The figure shows three views and two pictorial views of one solid part (mm, origin at its lowest corner). Answer the questions. Coordinates: 2 decimals unless noted, no trailing zeros. Order: outer loops, then holes, each group sorted by start corner. A loop starts at its lowest first (then second) coordinate and runs counter-clockwise, first axis right, second up. Notation, with made-up numbers: (69.5, -25) -> (124.5, -25) arc R25 ccw to (124.5, 7) -> close; hole circle Ø2 at (-33.75, -26.5). An arc over 180 degrees is marked (long way). Return JSON: item names as keys, results as strings.
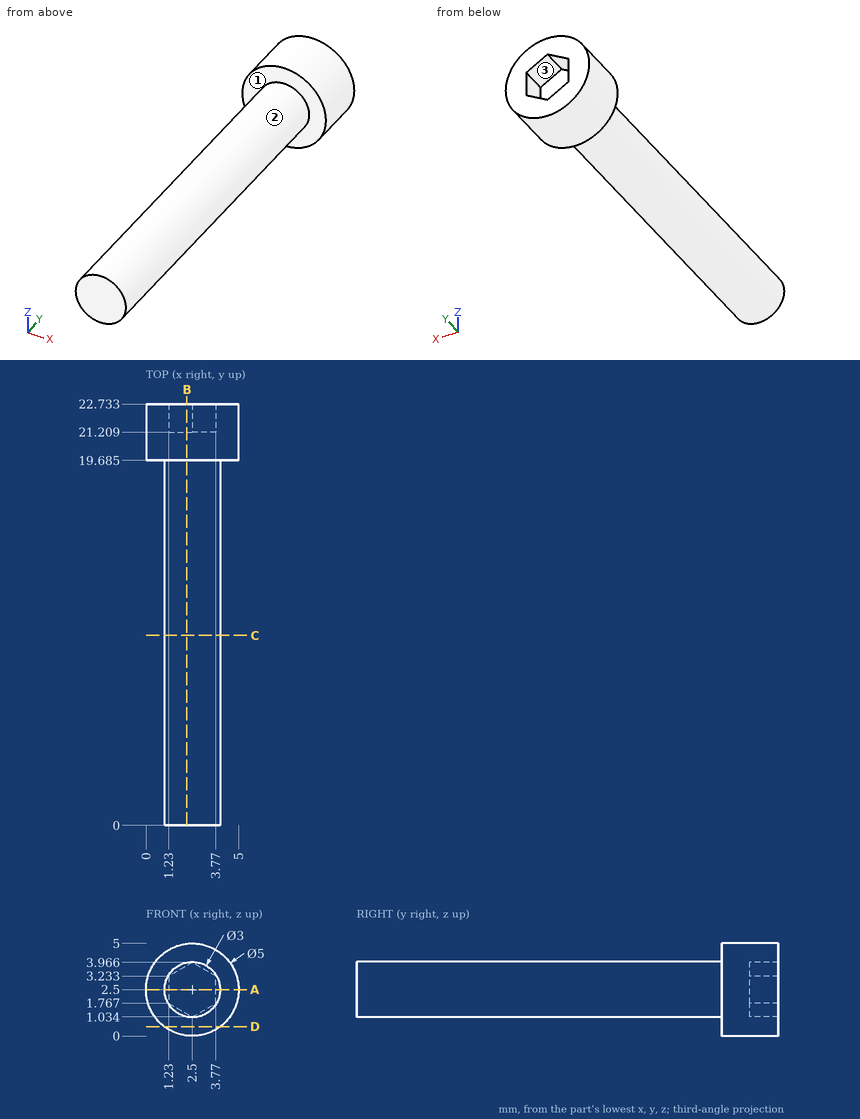
Item 1: The part is cut by section B-B on x = 2.2. Determine the outline of the cut face in (y, z) (1 decimal).
Answer list:
{"outline": "(0, 1) -> (19.7, 1) -> (19.7, 0) -> (22.7, 0) -> (22.7, 1.2) -> (21.2, 1.2) -> (21.2, 3.8) -> (22.7, 3.8) -> (22.7, 5) -> (19.7, 5) -> (19.7, 4) -> (0, 4) -> close"}
Item 2: The part is cut by section D-D on z = 0.5. Determine the outline of the cut face in (x, y) (1 decimal).
Answer list:
{"outline": "(1, 19.7) -> (4, 19.7) -> (4, 22.7) -> (1, 22.7) -> close"}
Item 3: Find the intervals of material crossed by probe 1 along Y at (x, z) = (4.1, 3.15) (1 decimal); probe 2 along X at (y, z) = (18, 1.7); probe 3 along Y at (x, z) = (2.45, 2.05), in increasing order.
Answer list:
{"probe 1": "19.7 to 22.7", "probe 2": "1.23 to 3.77", "probe 3": "0 to 21.21"}
Item 4: The part is cut by section A-A on z = 2.5. Determine the outline of the cut face in (x, y) (1 decimal).
Answer list:
{"outline": "(0, 19.7) -> (1, 19.7) -> (1, 0) -> (4, 0) -> (4, 19.7) -> (5, 19.7) -> (5, 22.7) -> (3.8, 22.7) -> (3.8, 21.2) -> (1.2, 21.2) -> (1.2, 22.7) -> (0, 22.7) -> close"}
Item 5: Flat-ended cylindrical pins translate along their axes: pin 1 (1 mm diameter, centred on y = 8.5, z = 4, fed in from +X); pin 2 (1 mm diameter, centred on x = 2.5, y = 16, fed in from +Z); pin 3 (2 mm diameter, centred on y = 5, z = 1, fed in from +X) (1 decimal). Find the tip coordinate at first contact, or state that the pin passes through.
Answer list:
{"pin 1": "x = 3.62", "pin 2": "z = 4", "pin 3": "x = 3.9"}
Item 6: The part is cut by section C-C on y = 10.25. Determine the outline of the cut face in (x, z).
Answer list:
{"outline": "circle Ø3 at (2.5, 2.5)"}
Item 7: Determine the mould class of the marked faces 1, 2 and 3 for opening direction Z: pulls with the +Z half, pulls with the -Z half, needs draft (parallel to the pull), parting line crosses it, or undercut.
Answer list:
{"face 1": "needs draft", "face 2": "parting line crosses it", "face 3": "undercut"}
